from build123d import *

# Parameters (mm, degrees)
SKETCH_1_W          = 30
SKETCH_1_H          = 30
EXTRUDE_1_DEPTH     = 40
SKETCH_2_W          = 30
SKETCH_2_H          = 10.165772452
EXTRUDE_2_DEPTH     = 60
SKETCH_3_R          = 12
EXTRUDE_3_DEPTH     = 5
SKETCH_4_R          = 9
EXTRUDE_4_DEPTH     = 5
SKETCH_16_R         = 9
CUT_EXTRUDE_1_DEPTH = 15


with BuildPart() as part:
    # Эскиз1 → Бобышка-Вытянуть1 (new body)
    with BuildSketch(Plane(origin=(0, 0, 0), x_dir=(0, 0, -1), z_dir=(1, 0, 0))):
        with Locations((-24.657846844, 7.360988518)):
            Rectangle(SKETCH_1_W, SKETCH_1_H)
    extrude(amount=EXTRUDE_1_DEPTH)

    # Эскиз2 → Бобышка-Вытянуть2 (add)
    with BuildSketch(Plane(origin=(40, 0, 0), x_dir=(0, 0, -1), z_dir=(1, 0, 0))):
        with Locations((-24.657846844, 17.278102292)):
            Rectangle(SKETCH_2_W, SKETCH_2_H)
    extrude(amount=EXTRUDE_2_DEPTH)

    # Эскиз3 → Бобышка-Вытянуть3 (add)
    with BuildSketch(Plane.XZ.offset(-12.195216066)):
        with Locations(Location((85, 24.657846844, 0), (0, 0, 90))):
            Circle(SKETCH_3_R)
    extrude(amount=EXTRUDE_3_DEPTH)

    # Эскиз4 → Бобышка-Вытянуть4 (add)
    with BuildSketch(Plane.XZ.offset(-7.195216066)):
        with Locations(Location((85, 24.657846844, 0), (0, 0, 270))):
            Circle(SKETCH_4_R)
    extrude(amount=EXTRUDE_4_DEPTH)

    # Эскиз13 → Цековка для  болта с шестигранной головкой M51 (revolve, cut)
    with BuildSketch(Plane(origin=(40, 2.482471753, 24.681970174), x_dir=(0, 0, -1), z_dir=(0, 1, 0))):
        Polygon((0, 0), (0, 40), (2.75, 40), (2.75, 3.5), (6.119, 3.5), (6.119, 0.025), (6.144, 0), align=None)
    revolve(axis=Axis((46.35, 2.482471753, 24.681970174), (-1, 0, 0)), mode=Mode.SUBTRACT)

    # Эскиз16 → Вырез-Вытянуть1 (cut)
    with BuildSketch(Plane(origin=(0, 22.360988518, 0), x_dir=(1, 0, 0), z_dir=(0, 1, 0))):
        with Locations(Location((85, -24.657846844, 0), (0, 0, 90))):
            Circle(SKETCH_16_R)
    extrude(amount=-CUT_EXTRUDE_1_DEPTH, mode=Mode.SUBTRACT)


solid = part.part
Build history of the part. All positions in model axes, mm. A direction names the side the tool comes from. Round coordinates to 2 decimals unless told otherwise and drop trailing zeros. Loops run counter-clockwise (first coordinate to the right, second up) from the corner with the lowest first, then second, coordinate; pieces in that order, holes last. Notation, with made-up numbers: (87.5, 6.5) -> (135.5, 6.5) arc R15 cw to (135.5, 32.5) -> close; hole circle Ø1 at (68.25, 52.25). An arc over 180 degrees is marked (long way). One line per item, written item: value. Start each with the question number.
Q1. Cut at C-C on z = 35. List the corners of the cut face in (x, y), plus the area to 3 significant figures.
Q2. Cut at D-D on x = 55. List the corners of the cut face in (y, z), plus the area to 3 significant figures.
Q3. Probe line 1 along Z through (x, y) = (85, 16); line 2 along X through (y, z) = (11.5, 26); line 3 along X through (y, z) = (14.25, 24.5). List the from-to ranges inside material, lowest first.
Q4. Cut at B-B on x = 17. List the corners of the cut face in (y, z), plus the area to 3 significant figures.
Q5. Two-plate mould, pull along Y, no slides. Class faces 5 (the face through (18.506, 3.536, 22.142)), 6 (the face through (38, 10, 39.658)), 7 (the face through (20, -7.639, 25)), 8 (the face through (36.5, 3.8, 27.3)): released by +Y, released by -Y, zero draft, split by the parting line, or undercut.
Q6. 3-axis set-ups, long thin cutter, end or side, ignore diameter. For faces 1 (the face through (92.98, 14.97, 20.5)), 2 (the face through (77.02, 4.73, 20.5)), 3 (the face through (38.26, 4.83, 19.03)), 4 (the face through (40, 9, 25)): which of +Z, -Z, +X, -X, +Y, -Y reach the whole face in a straight line?
Q7. Cut at A-A on x = 85. List the corners of the cut face in (y, z).
Q8. Drop flat-ended pins along their axis: pin 1 Ø10 at (y, z) = (3, 20.5) entering from -X; pin 2 Ø14 at (y, z) = (2.48, 24.68) entering from +X; pin 3 Ø14.5 at (x, z) = (85, 24.66) entering from -Y; pin 4 Ø3 at (x, y) = (70.5, 8.5) entering from -Z. Give the stop position or say it passes through.
Computed:
1. outline: (0, -7.64) -> (40, -7.64) -> (40, 12.2) -> (78.91, 12.2) -> (78.91, 7.2) -> (91.09, 7.2) -> (91.09, 12.2) -> (100, 12.2) -> (100, 22.36) -> (0, 22.36) -> close
1. area: 1,870 mm²
2. outline: (12.2, 9.66) -> (22.36, 9.66) -> (22.36, 39.66) -> (12.2, 39.66) -> close
2. area: 305 mm²
3. line 1: 9.66 to 15.66, 33.66 to 39.66
3. line 2: 0 to 40, 73.08 to 76.1, 93.9 to 96.92
3. line 3: 0 to 76, 94 to 100
4. outline: (-7.64, 9.66) -> (22.36, 9.66) -> (22.36, 39.66) -> (-7.64, 39.66) -> close; hole circle Ø5.5 at (2.48, 24.68)
4. area: 876 mm²
5. face 5: undercut
5. face 6: zero draft
5. face 7: released by -Y
5. face 8: undercut
6. face 1: +Y
6. face 2: -Y
6. face 3: none
6. face 4: +Z, -Z, -Y
7. outline: (2.2, 15.66) -> (7.2, 15.66) -> (7.2, 12.66) -> (12.2, 12.66) -> (12.2, 9.66) -> (22.36, 9.66) -> (22.36, 15.66) -> (7.36, 15.66) -> (7.36, 33.66) -> (22.36, 33.66) -> (22.36, 39.66) -> (12.2, 39.66) -> (12.2, 36.66) -> (7.2, 36.66) -> (7.2, 33.66) -> (2.2, 33.66) -> close
8. pin 1: x = 0
8. pin 2: x = 97
8. pin 3: y = 2.2
8. pin 4: through
